```python
from build123d import *

# Parameters (mm, degrees)
F0_W     = 533.4
F0_H     = 127
F1_DEPTH = 19.05
F2_W     = 533.4
F2_H     = 19.05
F3_DEPTH = 6.35
F4_R     = 1.5875
F5_DEPTH = 19.051


with BuildPart() as f1:
    # F0 (on Right) → F1 (new body)
    with BuildSketch(Plane.YZ):
        with Locations((266.7, -63.5)):
            Rectangle(F0_W, F0_H)
    extrude(amount=-F1_DEPTH)

    # F2 (on Right) → F3 (cut)
    with BuildSketch(Plane.YZ):
        with Locations((266.7, -111.125)):
            Rectangle(F2_W, F2_H)
    extrude(amount=-F3_DEPTH, mode=Mode.SUBTRACT)

    # F4 (on Right) → F5 (cut, through all)
    with BuildSketch(Plane.YZ):
        with Locations((63.5, -111.125)):
            Circle(F4_R)
        with Locations((165.1, -111.125)):
            Circle(F4_R)
        with Locations((266.7, -111.125)):
            Circle(F4_R)
        with Locations((368.3, -111.125)):
            Circle(F4_R)
        with Locations((469.9, -111.125)):
            Circle(F4_R)
    extrude(amount=-F5_DEPTH, mode=Mode.SUBTRACT)


solid = f1.part
```
Verification items for the finished model (mm, model axes). Round coordinates to 2 decimals unless told otherwise and drop trailing zeros. Order: outer loops, then holes, each group sorted by start corner. A loop starts at its lowest first (then second) coordinate and runs counter-clockwise, first axis right, second up. Notation, with made-up numbers: (11, 62.5) - (30, 62.5) arc R30 cw to (30, 93.5) - close; hole circle Ø9 at (29, -10.75). An arc over 180 degrees is marked (long way). Use CSV: the item, a comma, the result in double quotes.
(1) Thickness scan on probe 1 along Z at (x, y) = (-14.75, 266.7); probe 2 along Z at (x, y) = (-5, 468); probe 3 along X at (y, z) = (174, -111). Record the ranges inside material, lowest first. Write a range as from..to.
Entries:
probe 1,"-127..-112.71, -109.54..0"
probe 2,"-127..-120.65, -101.6..0"
probe 3,"-19.05..-6.35"
(2) Mould release check, pull along Z, two halves, no side actions. Record for faces 1 (the face through (0, 263, -50)), 2 (the face through (-9, 263, -127)), 3 (the face through (-9, 263, 0)), 4 (the face through (-6.35, 263, -111)): released by +Z, released by -Z, zero draft, split by the parting line, or undercut.
Entries:
face 1,"zero draft"
face 2,"released by -Z"
face 3,"released by +Z"
face 4,"undercut"
(3) Gauge pin test, flat end, axial feed: pin 1 Ø4 at (y, z) = (469.9, -111.125) entering from +X. Record the tip position at first contact, or that the pin passes through.
Entries:
pin 1,"x = -6.35"
(4) Section check A-A on y = 79. Record the boundary of the cut face in (x, z), and give its area (3 significant figures).
Entries:
outline,"(-19.05, -127) - (0, -127) - (0, -120.65) - (-6.35, -120.65) - (-6.35, -101.6) - (0, -101.6) - (0, 0) - (-19.05, 0) - close"
area,"2,300 mm^2"
